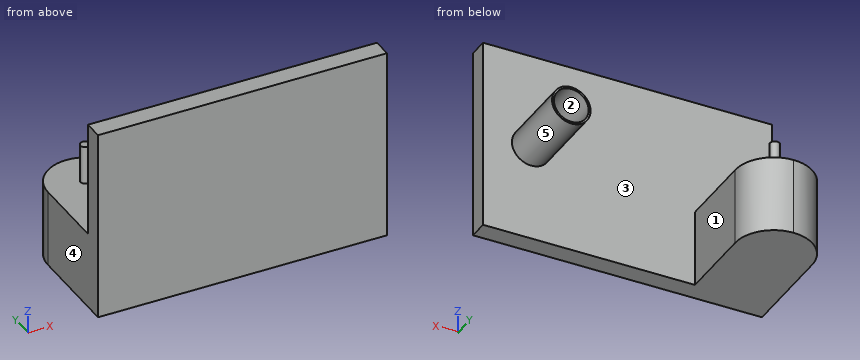
from build123d import *

# Parameters (mm, degrees)
SKETCH1_W           = 150
SKETCH1_H           = 100
BOSS_EXTRUDE1_DEPTH = 10
SKETCH2_R           = 10
BOSS_EXTRUDE2_DEPTH = 40
SKETCH3_R           = 9
CUT_EXTRUDE2_DEPTH  = 40
SKETCH4_W           = 40
SKETCH4_H           = 40
BOSS_EXTRUDE3_DEPTH = 60
CUT_EXTRUDE3_DEPTH  = 50
CUT_EXTRUDE4_DEPTH  = 50
SKETCH8_R           = 2.5
BOSS_EXTRUDE5_DEPTH = 20


with BuildPart() as part:
    # Sketch1 → Boss-Extrude1 (new body)
    with BuildSketch(Plane(origin=(0, 0, 0), x_dir=(1, 0, 0), z_dir=(0, 1, 0))):
        Rectangle(SKETCH1_W, SKETCH1_H)
    extrude(amount=BOSS_EXTRUDE1_DEPTH)

    # Sketch2 → Boss-Extrude2 (add)
    with BuildSketch(Plane(origin=(0, 10, 0), x_dir=(1, 0, 0), z_dir=(0, 1, 0))):
        with Locations(Location((50, 0, 0), (0, 0, 90))):
            Circle(SKETCH2_R)
    extrude(amount=BOSS_EXTRUDE2_DEPTH)

    # Sketch3 → Cut-Extrude2 (cut)
    with BuildSketch(Plane(origin=(0, 50, 0), x_dir=(1, 0, 0), z_dir=(0, 1, 0))):
        with Locations(Location((50, 0, 0), (0, 0, 270))):
            Circle(SKETCH3_R)
    extrude(amount=-CUT_EXTRUDE2_DEPTH, mode=Mode.SUBTRACT)

    # Sketch4 → Boss-Extrude3 (add)
    with BuildSketch(Plane(origin=(0, 10, 0), x_dir=(1, 0, 0), z_dir=(0, 1, 0))):
        with Locations((-55, 30)):
            Rectangle(SKETCH4_W, SKETCH4_H)
    extrude(amount=BOSS_EXTRUDE3_DEPTH)

    # Sketch6 → Cut-Extrude3 (cut)
    with BuildSketch(Plane.XY.offset(-10)):
        with BuildLine():
            Line((-75, 50), (-75, 70))
            Line((-75, 70), (-55, 70))
            ThreePointArc((-55, 70), (-69.142135624, 64.142135624), (-75, 50))
        make_face()
    extrude(amount=-CUT_EXTRUDE3_DEPTH, mode=Mode.SUBTRACT)

    # Sketch7 → Cut-Extrude4 (cut)
    with BuildSketch(Plane.XY.offset(-10)):
        with BuildLine():
            Line((-55, 70), (-35, 70))
            Line((-35, 70), (-35, 50))
            ThreePointArc((-35, 50), (-40.857864376, 64.142135624), (-55, 70))
        make_face()
    extrude(amount=-CUT_EXTRUDE4_DEPTH, mode=Mode.SUBTRACT)

    # Sketch8 → Boss-Extrude5 (add)
    with BuildSketch(Plane.XY.offset(-10)):
        with Locations(Location((-55.353289102, 50.491778343, 0), (0, 0, 180))):
            Circle(SKETCH8_R)
    extrude(amount=BOSS_EXTRUDE5_DEPTH)


solid = part.part
Geometry: final body of the model. Coordinates: model frame, mm. Face numbers are marked on the shaded views. A direction names the side the tool comes from. Give positions to 0.01 mm unless a question says otherwise; leave off trailing zeros. Order: outer loops, then holes, each group sorted by start corner. A loop starts at its lowest first (then second) coordinate and runs counter-clockwise, first axis right, second up. Notation, with made-up numbers: (27.25, 5.5) -> (32.25, 5.5) arc R23 cw to (32.25, 41.5) -> close; hole circle Ø10 at (78.25, -2). An arc over 180 degrees is marked (long way). Write each question's results on one line, items separated by ' | '.
1) Set-up query: the marked faces 4 and 5. Return all of +Z, -Z, +X, -X, +Y, -Y with unobstructed straight access to the full face (end or side cutting, diameter ignored); none if empty.
Geometry says:
face 4: +Z, -Z, -X, +Y, -Y | face 5: +Y
2) First-contact query: pin 1 Ø12 at (x, y) = (-61, 40.5) entering from +Z; pin 2 Ø6 at (x, z) = (50, 4) entering from +Y; pin 3 Ø1.5 at (x, y) = (57.5, 28) entering from -Z; pin 4 Ø12 at (x, y) = (-27, 31) entering from +Z. Flat tips, straight axial feed; report the tip coordinate or a pass-through.
Geometry says:
pin 1: stops at z = -10 | pin 2: stops at y = 10 | pin 3: stops at z = -7.38 | pin 4: passes through
3) Cut plane A-A (y = 36). Output: boundary loops of the cut face in (x, z).
Geometry says:
outline: (-75, -50) -> (-35, -50) -> (-35, -10) -> (-75, -10) -> close; circle Ø20 at (50, 0); hole circle Ø18 at (50, 0)
4) Cut plane C-C (z = -15). Output: boundary loops of the cut face in (x, y).
Geometry says:
outline: (-75, 0) -> (75, 0) -> (75, 10) -> (-35, 10) -> (-35, 50) arc R20 ccw to (-75, 50) -> close
5) Cut plane D-D (z = 2.5). Output: boundary loops of the cut face in (x, y), and give its area (3 significant figures).
Geometry says:
outline: (-75, 0) -> (75, 0) -> (75, 10) -> (59.68, 10) -> (59.68, 50) -> (58.65, 50) -> (58.65, 10) -> (41.35, 10) -> (41.35, 50) -> (40.32, 50) -> (40.32, 10) -> (-75, 10) -> close; circle Ø5 at (-55.35, 50.49) | area: 1,600 mm²
6) Cut plane B-B (x = 50). Output: boundary loops of the cut face in (y, z).
Geometry says:
outline: (0, -50) -> (10, -50) -> (10, -10) -> (50, -10) -> (50, -9) -> (10, -9) -> (10, 9) -> (50, 9) -> (50, 10) -> (10, 10) -> (10, 50) -> (0, 50) -> close
7) Line query: line 1 along X through (y, z) = (40, 0); line 2 along Y through (x, z) = (3, -18.5); line 3 along Z through (x, y) = (-38.5, 39). Output: solid intervals per line, ascending.
Geometry says:
line 1: x = 40 to 41, 59 to 60 | line 2: y = 0 to 10 | line 3: z = -50 to -10
8) Draft query along X for the marked faces 1, 2 and 3. Return one class per face: released by +X, released by -X, zero draft, split by the parting line, or undercut.
Geometry says:
face 1: released by +X | face 2: undercut | face 3: zero draft
